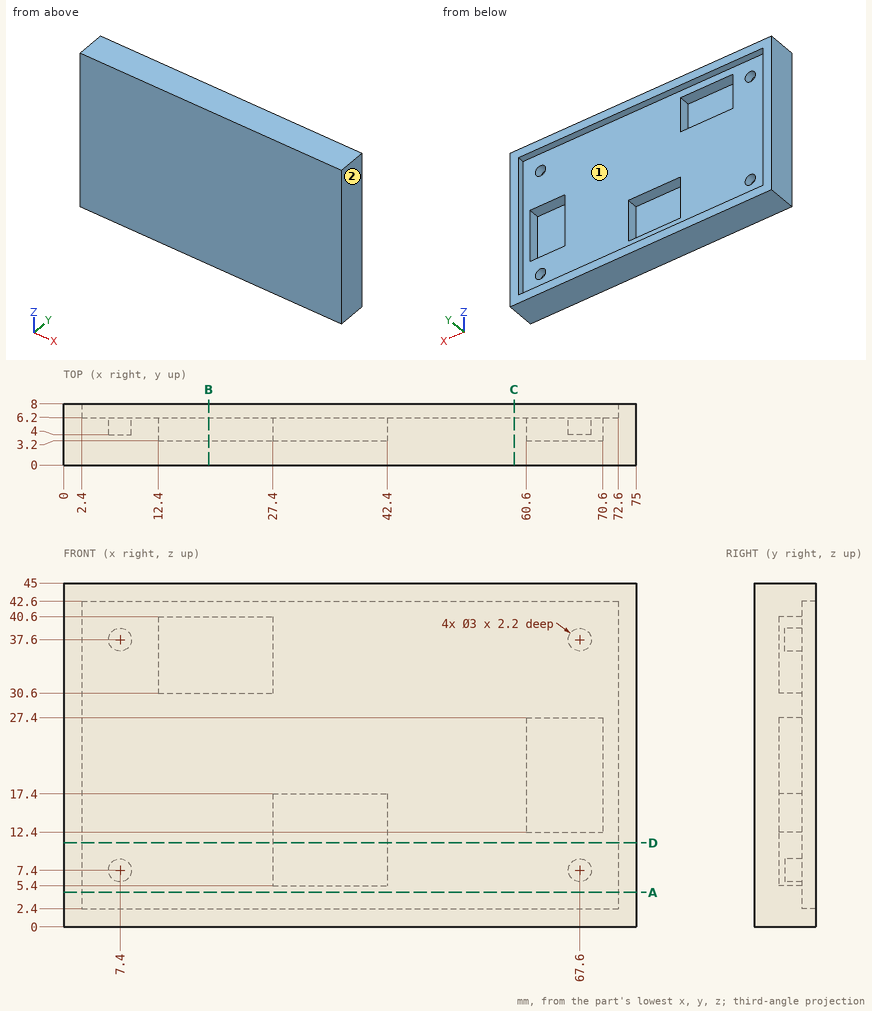
Drawing for the job (mm, zero at the part's lowest x, y, z). A direction names the side the tool comes from. Round coordinates to 2 decimals unless told otherwise and drop trailing zeros. Order: outer loops, then holes, each group sorted by start corner. A loop starts at its lowest first (then second) coordinate and runs counter-clockwise, first axis right, second up. Notation, with made-up numbers: (88, 76.25) -> (96, 76.25) arc R20 ccw to (96, 85.25) -> close; hole circle Ø1 at (51, 41.5). An arc over 180 degrees is marked (long way). Put each result on its own line as item: value.
Q1. Band-saw the part on D-D (z = 11). Give the cut face in (x, y), and give its area (3 significant figures).
From the geometry:
outline: (0, 0) -> (75, 0) -> (75, 8) -> (72.6, 8) -> (72.6, 6.2) -> (42.4, 6.2) -> (42.4, 3.2) -> (27.4, 3.2) -> (27.4, 6.2) -> (2.4, 6.2) -> (2.4, 8) -> (0, 8) -> close
area: 429 mm2
Q2. Band-saw the part on A-A (z = 4.5). Give the cut face in (x, y), and give its area (3 significant figures).
From the geometry:
outline: (0, 0) -> (75, 0) -> (75, 8) -> (72.6, 8) -> (72.6, 6.2) -> (2.4, 6.2) -> (2.4, 8) -> (0, 8) -> close
area: 474 mm2
Q3. Pin check, flat tips, straight feed: pin 1 Ø5 at (x, z) = (67, 19) entering from +Y; pin 2 Ø11 at (x, z) = (17, 35.5) entering from +Y. Stop position of each tip, or through.
From the geometry:
pin 1: stops at y = 3.2
pin 2: stops at y = 6.2
Q4. Band-saw the part on C-C (x = 59). Give the cut face in (y, z), and give its area (3 significant figures).
From the geometry:
outline: (0, 0) -> (8, 0) -> (8, 2.4) -> (6.2, 2.4) -> (6.2, 42.6) -> (8, 42.6) -> (8, 45) -> (0, 45) -> close
area: 288 mm2
Q5. Band-saw the part on B-B (x = 19). Give the cut face in (y, z).
From the geometry:
outline: (0, 0) -> (8, 0) -> (8, 2.4) -> (6.2, 2.4) -> (6.2, 30.6) -> (3.2, 30.6) -> (3.2, 40.6) -> (6.2, 40.6) -> (6.2, 42.6) -> (8, 42.6) -> (8, 45) -> (0, 45) -> close
Q6. Wall check: line 1 (X direction, y = 4.9, z = 37.6); line 2 (X direction, y = 5.1, z = 7.4); line 3 (X direction, y = 3.5, z = 10.5). Give the ranges that are in metal, low to high. Write a range as [from, to].
From the geometry:
line 1: x = [0, 5.9], [8.9, 12.4], [27.4, 66.1], [69.1, 75]
line 2: x = [0, 5.9], [8.9, 27.4], [42.4, 66.1], [69.1, 75]
line 3: x = [0, 27.4], [42.4, 75]
Q7. Tool access for the marked faces 1 and 2: list every direction of +Z, -Z, +X, -X, +Y, -Y with a clear straight run to the whole face (end or side of a thin tool).
From the geometry:
face 1: +Y
face 2: +Z, -Z, +X, +Y, -Y
